```python
from build123d import *

# Parameters (mm, degrees)
FILLET1_R          = 2
SKETCH2_R          = 1.5
CUT_EXTRUDE1_DEPTH = 18


with BuildPart() as part:
    # Sketch1 → Revolve1 (revolve)
    with BuildSketch(Plane.XY):
        Polygon((0, 0), (0, 25), (-2.744112853, 25), (-2.744112853, 8.642091449), (-6.244112853, 8.642091449), (-6.244112853, 7.755870593), (-5, 7.343117412), (-5, 0), align=None)
    revolve(axis=Axis((0, 0, 0), (0, 1, 0)))

    # Fillet1
    fillet1_edges = [part.edges().sort_by_distance(p)[0] for p in [
        (2.744112853, 25, 0),
    ]]
    fillet(fillet1_edges, radius=FILLET1_R)

    # Sketch2 → Cut-Extrude1 (cut)
    with BuildSketch(Plane.XZ):
        Circle(SKETCH2_R)
    extrude(amount=-CUT_EXTRUDE1_DEPTH, mode=Mode.SUBTRACT)


solid = part.part
```
The model under review builds one solid part; all positions refer to its coordinate system, in mm. A direction names the side the tool comes from. Round coordinates to 2 decimals unless told otherwise and drop trailing zeros. Write each loop counter-clockwise with the first axis right and the second up, starting at its lowest first coordinate (ties: lowest second). Pieces come first, ordered by that corner, then holes. Notation, with made-up numbers: (12.25, 48) - (63.25, 48) arc R24 ccw to (63.25, 86) - close; hole circle Ø1 at (34.25, 78.25). An arc over 180 degrees is marked (long way). Answer as CSV lines item,"result". Start each with the question number.
(1) To check wall thickness, follow line 1 (Z direction, x = 0, y = 13.75); line 2 (Y direction, x = 0, z = -3); line 3 (Z direction, x = 0, y = 4.25). State the ranges of each line that lie inside material, in increasing order.
(2) Draft analysis for pull direction X (two halves, no side actions). For faces 1 (the cylindrical face through (1.08, 3.62, -4.88)), 2 (the flat face through (3, 8.642, -1)), 3 (the cylindrical face through (-1.5, 8.87, 0.07)), state which applies: pulls with the +X half, pulls with the -X half, needs draft (parallel to the pull), parting line crosses it, or undercut.
(3) We need section B-B on y = 21. State the section outline as (x, z) points, plus the area to 3 significant figures.
(4) For faces 4 (the cylindrical face through (0.59, 15.72, -2.68)), 5 (the flat face through (1.2, 0, 1.2)), 6 (the flat face through (0, 18, 0)), list the 3-axis set-ups (+Z, -Z, +X, -X, +Y, -Y) from which the entire face can be reached by the end or side of a thin tool; tool diameter is ignored.
(5) We need section A-A on y = 16.5. State the section outline as (x, z) points.
(6) For pin 1 Ø1 at (x, z) = (1.5, -3.5) entering from +Y; pin 2 Ø6 at (x, y) = (2.5, 18.5) entering from +Z; pin 3 Ø1.5 at (x, z) = (-0.5, -0.5) entering from -Y, all flat-tipped, find the tip position at first contact; note any pin that passes through.
(7) We need section C-C on y = 2.5. State the section outline as (x, z) points, plus the area to 3 significant figures.
Worked answers:
1,line 1,"-2.74 to -1.5, 1.5 to 2.74"
1,line 2,"0 to 8.64"
1,line 3,"-5 to -1.5, 1.5 to 5"
2,face 1,"parting line crosses it"
2,face 2,"needs draft"
2,face 3,"undercut"
3,outline,"circle Ø5.49 at (0, 0)"
3,area,"23.7 mm²"
4,face 4,"+Y"
4,face 5,"+Z, -Z, +X, -X, -Y"
4,face 6,"-Y"
5,outline,"circle Ø5.49 at (0, 0); hole circle Ø3 at (0, 0)"
6,pin 1,"y = 8.64"
6,pin 2,"z = 2.74"
6,pin 3,"y = 18"
7,outline,"circle Ø10 at (0, 0); hole circle Ø3 at (0, 0)"
7,area,"71.5 mm²"
